Can you work these out from the drawing? Everything is in mm from the part's minimum corner. A direction names the side the tool comes from. Coordinates: 2 decimals unless noted, no trailing zeros. Write each loop counter-clockwise with the first axis right and the second up, starting at its lowest first coordinate (ties: lowest second). Pieces come first, ordered by that corner, then holes. Notation, with made-up numbers: (80, 17) -> (112, 17) arc R15 ccw to (112, 32) -> close; hole circle Ø8 at (37, -7). An arc over 180 degrees is marked (long way). Use a Markdown table: item, result. Add a question column.
Item 1: Imagine slicing it at C-C, the plane y = 45. Write out the boundary of the cut face in (x, z), and give its area (3 significant figures).
Item 2: If I drill on line 1 along Z through (x, y) = (27, 40.5); line 2 along Z through (x, y) = (35.5, 23); line 3 along Y through (x, z) = (31.5, 28) (1 decimal), over which ranges is the centre line in solid material (lowest first)? Write a range as from..to.
Item 3: Imagine slicing it at B-B, the plane x = 12. Write out the boundary of the cut face in (y, z).
Item 4: If we mould it in two halves opening along X, with no side actions, what happens to the marked faces 1, 2 and 3? For each: pulls with the +X half, pulls with the -X half, needs draft (parallel to the pull), parting line crosses it, or undercut.
Item 5: Imagine slicing it at D-D, the plane z = 34.5. Write out the boundary of the cut face in (x, y) (1 decimal).
Item 6: Imagine slicing it at A-A, the plane y = 29.5. Write out the boundary of the cut face in (x, z) (1 decimal).
Item 7: On a 3-axis mill with a long thin cutter (end or side, diameter ignored), from which of +Z, -Z, +X, -X, +Y, -Y can I reach the whole of each face in a straight line? I mean the marked faces 4 and 5. Say none if no direction works.
Item 8: Will this pin go through, and if not, where does the flat tip stop? pin 1 Ø5 at (x, y) = (52, 7.5) entering from +Z.
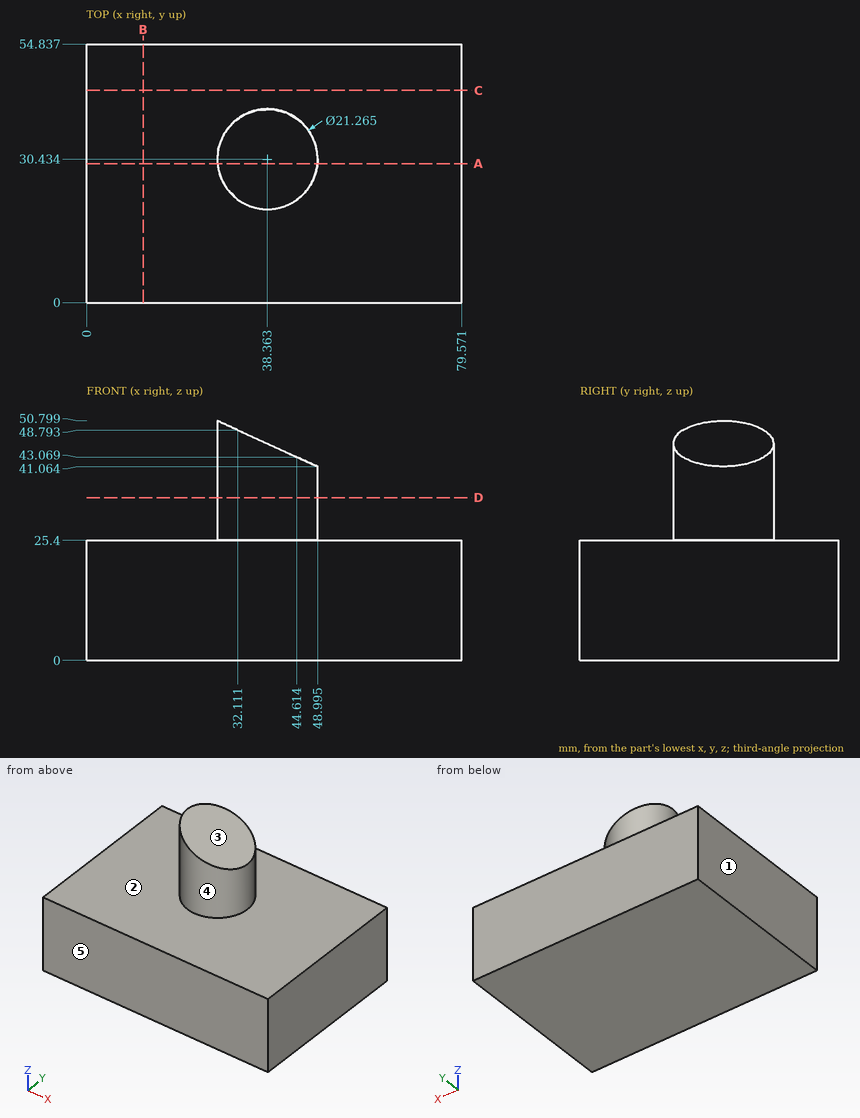
Ans:
| question | item | result |
|---|---|---|
| 1 | outline | (0, 0) -> (79.57, 0) -> (79.57, 25.4) -> (0, 25.4) -> close |
| 1 | area | 2,020 mm^2 |
| 2 | line 1 | z = 0..25.4 |
| 2 | line 2 | z = 0..47.24 |
| 2 | line 3 | y = 22.3..38.6 |
| 3 | outline | (0, 0) -> (54.84, 0) -> (54.84, 25.4) -> (0, 25.4) -> close |
| 4 | face 1 | pulls with the -X half |
| 4 | face 2 | needs draft |
| 4 | face 3 | pulls with the +X half |
| 5 | outline | circle Ø21.3 at (38.4, 30.4) |
| 6 | outline | (0, 0) -> (79.6, 0) -> (79.6, 25.4) -> (49, 25.4) -> (49, 41.1) -> (27.8, 50.8) -> (27.8, 25.4) -> (0, 25.4) -> close |
| 7 | face 4 | +Z |
| 7 | face 5 | +Z, -Z, +X, -X, -Y |
| 8 | pin 1 | stops at z = 25.4 |
